from build123d import *

# Parameters (mm, degrees)
F0_W     = 75
F0_H     = 75
F0_W_2   = 66
F0_H_2   = 66
F1_DEPTH = 2394
F2_R     = 30
F3_DEPTH = 9.5
F5_DEPTH = 3


with BuildPart() as f1:
    # F0 (on Top) → F1 (new body)
    with BuildSketch(Plane.XY):
        Rectangle(F0_W, F0_H)
        Rectangle(F0_W_2, F0_H_2, mode=Mode.SUBTRACT)
    extrude(amount=F1_DEPTH)

    # F2 (on Front) → F3 (join, symmetric)
    with BuildSketch(Plane.XZ):
        with BuildLine():
            Line((-50, 2494), (-50, 2344))
            Line((-50, 2344), (50, 2344))
            Line((50, 2344), (50, 2494))
            ThreePointArc((50, 2494), (0, 2544), (-50, 2494))
        make_face()
        with Locations((0, 2494)):
            Circle(F2_R, mode=Mode.SUBTRACT)
    extrude(amount=F3_DEPTH, both=True)

    # F4 (on Front) → F5 (join, symmetric)
    with BuildSketch(Plane.XZ):
        Polygon((-112.5, 0), (-37.5, 0), (-37.5, 75), align=None)
    extrude(amount=F5_DEPTH, both=True)


solid = f1.part
The model under review builds one solid part; all positions refer to its coordinate system, in mm. A direction names the side the tool comes from. Round coordinates to 2 decimals unless told otherwise and drop trailing zeros. Loops run counter-clockwise (first coordinate to the right, second up) from the corner with the lowest first, then second, coordinate; pieces in that order, holes last. Notation, with made-up numbers: M 49,70 L 56,70 A25 cw 56,95 Z; hole C 5.5,85.5 d9. An arc over 180 degrees is marked long. Answer as a JSON object with one key per item and string values.
Item 1: For line 1 along X through (y, z) = (-2, 2494); line 2 along X through (y, z) = (8.5, 696), list the stretches that pass through material, from the lowest coordinate up.
Check sheet entries:
{"line 1": "-50 to -30, 30 to 50", "line 2": "-37.5 to -33, 33 to 37.5"}
Item 2: We need section C-C, the plane y = 21. State the section outline as (x, z) points, and give its area (3 significant figures).
Check sheet entries:
{"outline": "M -37.5,0 L -33,0 L -33,2394 L -37.5,2394 Z; M 33,0 L 37.5,0 L 37.5,2394 L 33,2394 Z", "area": "21,500 mm2"}
Item 3: Tool access review of faces 1 (the face through (-74.5, 0, 38)), 2 (the face through (-59, 3, 21)), 3 (the face through (0, -33, 1180)): name each direction out of +Z, -Z, +X, -X, +Y, -Y from which nothing blocks a thin tool from reaching the whole face with its end or side.
Check sheet entries:
{"face 1": "-X, +Y, -Y", "face 2": "-Z, -X, +Y", "face 3": "+Z, -Z"}
Item 4: Clearance check with flat-ended pins moving along their axes: P1, Ø4, axis at x = 44, y = -2.5, coming from the -Z side; P2, Ø4, axis at y = 18, z = 1484.5, coming from the +X side; P3, Ø1, axis at y = -17.5, z = 739.5, coming from the -X side. State where each tip first meets the part, or that it passes through.
Check sheet entries:
{"P1": "z = 2344", "P2": "x = 37.5", "P3": "x = -37.5"}
Item 5: We need section A-A, the plane z = 600.5. State the section outline as (x, y) points.
Check sheet entries:
{"outline": "M -37.5,-37.5 L 37.5,-37.5 L 37.5,37.5 L -37.5,37.5 Z; hole M -33,-33 L 33,-33 L 33,33 L -33,33 Z"}
Item 6: We need section B-B, the plane x = 0. State the section outline as (y, z) points.
Check sheet entries:
{"outline": "M -37.5,0 L -33,0 L -33,2394 L -37.5,2394 Z; M -9.5,2344 L 9.5,2344 L 9.5,2464 L -9.5,2464 Z; M -9.5,2524 L 9.5,2524 L 9.5,2544 L -9.5,2544 Z; M 33,0 L 37.5,0 L 37.5,2394 L 33,2394 Z"}
Item 7: The part is to be moulded in two halves that separate along Y. For faces 4 (the face through (-1, -9.5, 2423)), 5 (the face through (-59, -3, 21)), 6 (the face through (33, 0, 1180)), 7 (the face through (1.099, -0.133, 2543.988)), say which applies: +Y half, -Y half, draft (parallel to the pull), parting line (faces both ways), or undercut.
Check sheet entries:
{"face 4": "undercut", "face 5": "-Y half", "face 6": "undercut", "face 7": "draft"}
